Build history of the part. All positions in model axes, mm. Face numbers are marked on the shaded views. A direction names the side the tool comes from. Give positions to 0.01 mm unless a question says otherwise; leave off trailing zeros. Write each loop counter-clockwise with the first axis right and the second up, starting at its lowest first coordinate (ties: lowest second). Pieces come first, ordered by that corner, then holes. Notation, with made-up numbers: (27.25, -32) -> (60.25, -32) arc R19 ccw to (60.25, 2) -> close; hole circle Ø9 at (76.5, 7.5). An arc over 180 degrees is marked (long way). Write item = value, one per line. Start each with the question number.
Q1. Saw through at B-B, the plane y = 5. List the corners of the cut face in (x, z).
Q2. Saw through at A-A, the plane z = 0. List the corners of the cut face in (x, y).
Q3. Saw through at C-C, the plane z = -10.5. List the corners of the cut face in (x, y), then the cut area to 3 significant figures.
Q4. Drop flat-ended pins along their axis: P1, Ø8.5, axis at y = 137.5, z = -6, coming from the -X side; P2, Ø5.5, axis at y = -127.5, z = 6, coming from the +X side; P3, Ø9, axis at y = -1, z = 6.5, coming from the +X side. Give the stop position or say it passes through.
Q5. Saw through at D-D, the plane x = 3.5. List the corners of the cut face in (y, z), then the cut area to 3 significant figures.
Q6. Mould opens along Y. For the marked faces 1, 2, 3 and 4 say: pulls with the +Y half, pulls with the -Y half, needs draft (parallel to the pull), parting line crosses it, or undercut.
Q7. Tool access for the marked faces 5, 6, 7, 8 and 9: list every direction of +Z, -Z, +X, -X, +Y, -Y with a clear straight run to the whole face (end or side of a thin tool).
Q8. Wall check: line 1 (Y direction, x = 8.5, z = 6.25); line 2 (X direction, y = -24.5, z = 5.75); line 3 (Y direction, x = 11.5, z = -12.5). Give the ranges that are in metal, low to high.
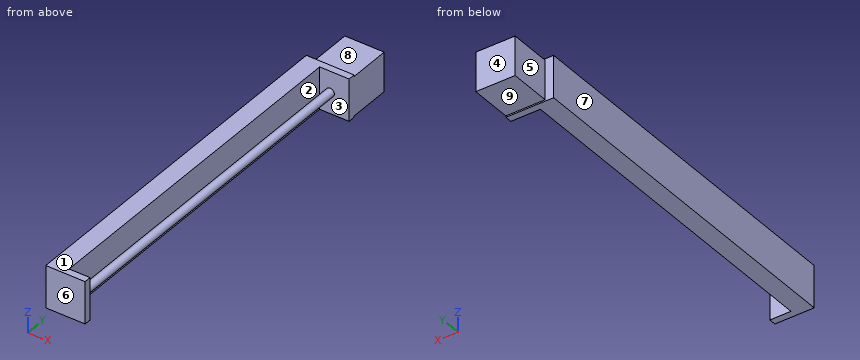
from build123d import *

# Parameters (mm, degrees)
SKETCH1_W           = 34
SKETCH1_H           = 5
SKETCH1_W_2         = 13
SKETCH1_H_2         = 250
BOSS_EXTRUDE1_DEPTH = 15
SKETCH1_3_W         = 28
SKETCH1_3_H         = 30
BOSS_EXTRUDE2_DEPTH = 14
SKETCH2_R           = 3
BOSS_EXTRUDE3_DEPTH = 250


with BuildPart() as part:
    # Sketch1 → Boss-Extrude1 (new, symmetric)
    with BuildSketch(Plane.XY):
        with Locations((0, 127.5)):
            Rectangle(SKETCH1_W, SKETCH1_H)
        with Locations((-10.5, 0)):
            Rectangle(SKETCH1_W_2, SKETCH1_H_2)
        Polygon((-4, -125), (-17, -125), (-17, -130), (11, -130), (11, -125), align=None)
    extrude(amount=BOSS_EXTRUDE1_DEPTH, both=True)

    # Sketch1<3> → Boss-Extrude2 (add, symmetric)
    with BuildSketch(Plane.XY):
        with Locations((3, 145)):
            Rectangle(SKETCH1_3_W, SKETCH1_3_H)
    extrude(amount=BOSS_EXTRUDE2_DEPTH, both=True)

    # Sketch2 → Boss-Extrude3 (add)
    with BuildSketch(Plane(origin=(0, -125, 0), x_dir=(1, 0, 0), z_dir=(0, 1, 0))):
        with Locations(Location((3.5, 0, 0), (0, 0, 90))):
            Circle(SKETCH2_R)
    extrude(amount=BOSS_EXTRUDE3_DEPTH)


solid = part.part
Report:
q1.outline = (-17, -15) -> (-4, -15) -> (-4, 15) -> (-17, 15) -> close; circle Ø6 at (3.5, 0)
q2.outline = (-17, -130) -> (11, -130) -> (11, -125) -> (6.5, -125) -> (6.5, 125) -> (17, 125) -> (17, 160) -> (-11, 160) -> (-11, 130) -> (-17, 130) -> close; hole (-4, -125) -> (0.5, -125) -> (0.5, 125) -> (-4, 125) -> close
q3.outline = (-17, -130) -> (11, -130) -> (11, -125) -> (-4, -125) -> (-4, 125) -> (17, 125) -> (17, 160) -> (-11, 160) -> (-11, 130) -> (-17, 130) -> close
q3.area = 4,400 mm2
q4.P1 = -11
q4.P2 = 11
q4.P3 = 5.74
q5.outline = (-130, -15) -> (-125, -15) -> (-125, -3) -> (125, -3) -> (125, -15) -> (130, -15) -> (130, -14) -> (160, -14) -> (160, 14) -> (130, 14) -> (130, 15) -> (125, 15) -> (125, 3) -> (-125, 3) -> (-125, 15) -> (-130, 15) -> close
q5.area = 2,640 mm2
q6.face_1 = needs draft
q6.face_2 = undercut
q6.face_3 = undercut
q6.face_4 = pulls with the +Y half
q7.face_5 = +Z, -Z, -X, +Y
q7.face_6 = +Z, -Z, +X, -X, -Y
q7.face_7 = +Z, -Z, -X, +Y, -Y
q7.face_8 = +Z, +X, -X, +Y
q7.face_9 = -Z, +X, -X, +Y
q8.line_1 = -130 to -125, 125 to 160
q8.line_2 = -17 to -4
q8.line_3 = 125 to 160
